Part model, mm, in its own coordinate system. Round coordinates to 2 decimals unless told otherwise and drop trailing zeros. Loops run counter-clockwise (first coordinate to the right, second up) from the corner with the lowest first, then second, coordinate; pieces in that order, holes last. Notation, with made-up numbers: M 69,22 L 118,22 A16 ccw 118,38 Z; hole C -20.75,-4 d4. An arc over 180 degrees is marked long. Put each result on its own line as item: value. Start each with the question number.
1) Slice it at A-A on z = 5. State how many separate pieces and enclosed holes the cut face has, then the cut area to 3 significant figures.
2) Probe line 1 along Z through (x, y) = (107.5, 87); line 2 along Y through (x, z) = (13, 5); line 3 along Y through (x, z) = (65, 9.75). List the from-to ranges inside material, lowest first.
3) Slice it at C-C on x = 64. Give the cut face in (y, z).
4) Drop flat-ended pins along their axis: pin 1 Ø4 at (x, y) = (13, -5) entering from -Z; pin 2 Ø5 at (y, z) = (113, 5) entering from -X; pin 3 Ø4 at (x, z) = (35, 2.5) entering from -Y; pin 4 Ø1 at (y, z) = (46.5, 6.5) entering from +X. Give the stop position or say it passes through.
5) Slice it at B-B on y = 17. Give the cut face in (x, z).
```python
from build123d import *

# Parameters (mm, degrees)
SKETCH1_R           = 1.75
BOSS_EXTRUDE1_DEPTH = 10
SKETCH2_R           = 1.5
CUT_EXTRUDE1_DEPTH  = 15


with BuildPart() as part:
    # Sketch1 → Boss-Extrude1 (new body)
    with BuildSketch(Plane.XY):
        Polygon((-125, 75), (-125, 50), (-75, 0), (-25, 0), (-25, -10), (25, -10), (25, 0), (75, 0), (125, 50), (125, 75), (115, 75), (115, 125), (125, 125), (125, 250), (-125, 250), (-125, 125), (-115, 125), (-115, 75), align=None)
        with Locations((-13, -5)):
            Circle(SKETCH1_R, mode=Mode.SUBTRACT)
        with Locations((13, -5)):
            Circle(SKETCH1_R, mode=Mode.SUBTRACT)
    extrude(amount=BOSS_EXTRUDE1_DEPTH)

    # Sketch2 → Cut-Extrude1 (cut)
    with BuildSketch(Plane(origin=(115, 0, 0), x_dir=(0, 0, -1), z_dir=(1, 0, 0))):
        with Locations(Location((-5, 113, 0), (0, 0, 90))):
            Circle(SKETCH2_R)
        with Locations(Location((-5, 87, 0), (0, 0, 90))):
            Circle(SKETCH2_R)
    cut_extrude1 = extrude(amount=-CUT_EXTRUDE1_DEPTH, mode=Mode.SUBTRACT)

    # Mirror1: Cut-Extrude1 across plane
    add(cut_extrude1.mirror(Plane(origin=(0, 0, 0), x_dir=(0, 0, 1), z_dir=(1, 0, 0))), mode=Mode.SUBTRACT)


solid = part.part
```
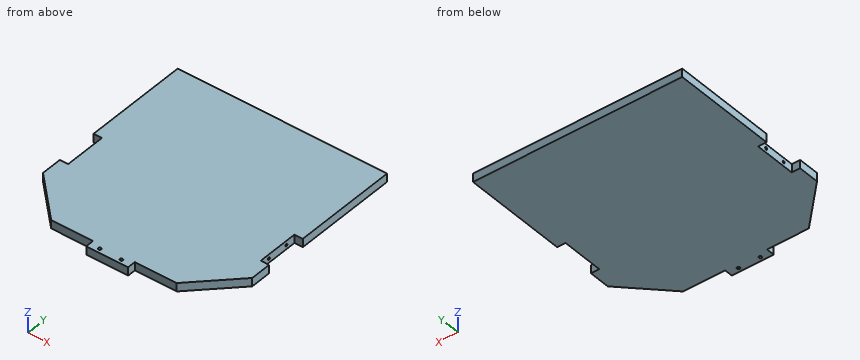
Recorded:
1. separate pieces: 1
1. enclosed holes: 2
1. area: 59,300 mm2
2. line 1: z = 0 to 3.5, 6.5 to 10
2. line 2: y = -10 to -6.75, -3.25 to 250
2. line 3: y = 0 to 250
3. outline: M 0,0 L 250,0 L 250,10 L 0,10 Z
4. pin 1: stops at z = 0
4. pin 2: stops at x = -115
4. pin 3: stops at y = 0
4. pin 4: stops at x = 122
5. outline: M -92,0 L 92,0 L 92,10 L -92,10 Z
